Could you check a few things on this drawing? It's one solid part, dimensions in mm from its lowest x, y, z. Coordinates: 2 decimals unless noted, no trailing zeros. Write each loop counter-clockwise with the first axis right and the second up, starting at its lowest first coordinate (ties: lowest second). Pieces come first, ordered by that corner, then holes.
Item 1: I'm going to push flat-ended pins straight in: P1, Ø1, axis at x = 8.5, y = 2.5, coming from the +Z side; P2, Ø1.5, axis at y = 1.5, z = 15, coming from the -X side. Where does each tip first touch, or does it pass through?
Item 2: I want a section at C-C (y = 0.65). Please give me the cut outline in (x, z).
Item 3: Please list where these lines run through material, in increasing order: line 1 (Z direction, x = 10.5, y = 1.6); line 2 (X direction, y = 1.3, z = 5.25); line 3 (Z direction, x = 6.5, y = 2.85).
Item 4: I want a section at B-B (y = 2.6). Please give me the cut outline in (x, z).
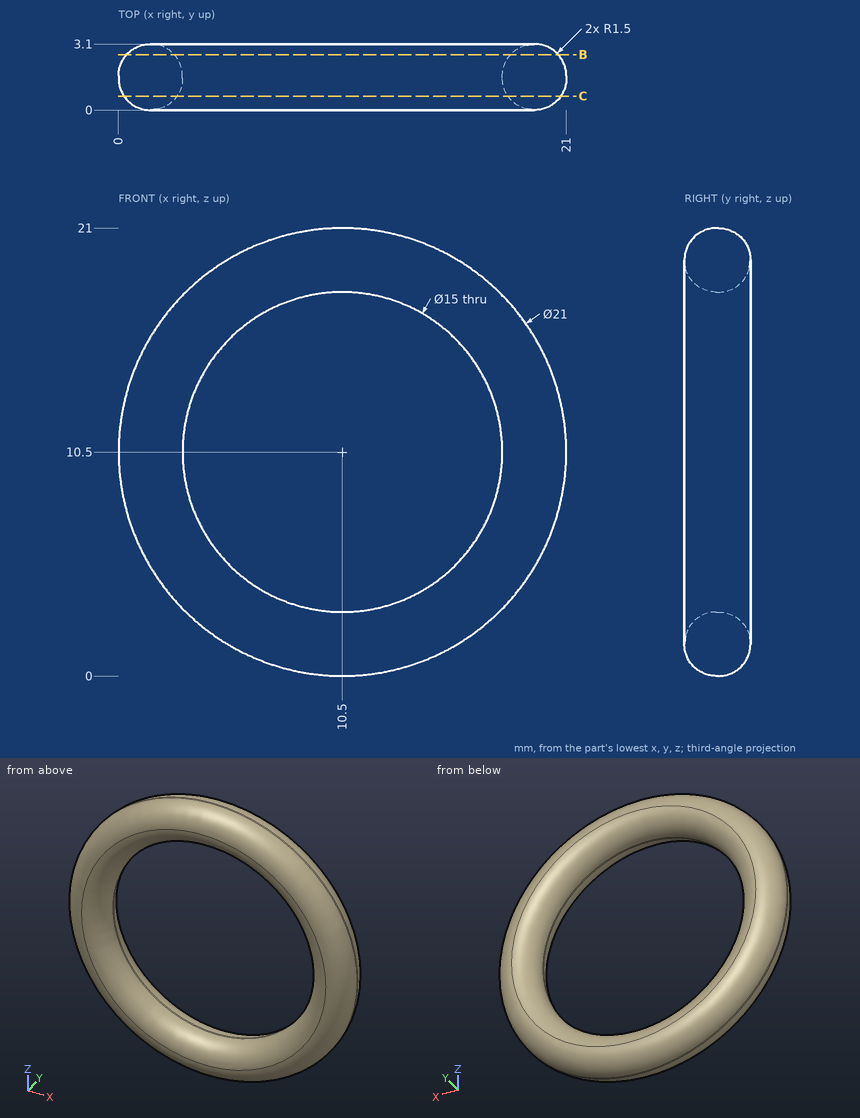
Answer:
1. P1: stops at z = 20.78
1. P2: stops at x = 0.69
2. outline: circle Ø20.47 at (10.5, 10.5); hole circle Ø15.53 at (10.5, 10.5)
3. line 1: z = 0 to 3, 18 to 21
3. line 2: x = 1.42 to 5.13, 15.87 to 19.58
3. line 3: z = 1.52 to 3.38, 17.62 to 19.48
4. outline: circle Ø20.24 at (10.5, 10.5); hole circle Ø15.76 at (10.5, 10.5)
